```python
from build123d import *

# Parameters (mm, degrees)
BASE_FLANGE1_DEPTH           = 2.65684
SKETCHED_BEND3_DEPTH         = 355.6
SKETCHED_BEND3_2_DEPTH       = 355.6
SKETCH10_R                   = 6.35
CUT_EXTRUDE2_DEPTH           = 2.65684
EDGE_FLANGE5_DEPTH           = 254
EDGE_FLANGE6_STRIP_W         = 16.97736
EDGE_FLANGE6_STRIP_H         = 2.65684
EDGE_FLANGE6_STRIP_CUT_DEPTH = 116.5225
EDGE_FLANGE6_DEPTH           = 116.5225
EDGE_FLANGE7_DEPTH           = 248.16816
SKETCH38_R                   = 2.032
CUT_EXTRUDE4_DEPTH           = 2.65684
SKETCH39_R                   = 2.032
CUT_EXTRUDE5_DEPTH           = 2.65684
SKETCH40_R                   = 6.35
CUT_EXTRUDE6_DEPTH           = 2.65684


# Read off the part's stored shape, not the designer's step: Sketched Bend3
# Sheet-metal steps are written as plain solids
with BuildPart() as part:
    # Sketch1 → Base-Flange1 (new body)
    with BuildSketch(Plane.XY):
        with BuildLine():
            Line((0, 0), (0, 254))
            Line((0, 254), (165.1, 254))
            ThreePointArc((165.1, 254), (177.8, 241.3), (190.5, 254))
            Line((190.5, 254), (355.6, 254))
            Line((355.6, 254), (355.6, 0))
            Line((355.6, 0), (355.6, -57.15))
            Line((355.6, -57.15), (0, -57.15))
            Line((0, -57.15), (0, 0))
        make_face()
    extrude(amount=-BASE_FLANGE1_DEPTH)

    # Sketched Bend3 outline → Sketched Bend3 (cut)
    with BuildSketch(Plane.YZ):
        with BuildLine():
            ThreePointArc((0, -2.65684), (-2.783367186, -1.949765838), (-4.891802611, 0))
            Line((-4.891802611, 0), (-57.15, 0))
            Line((-57.15, 0), (-57.15, -2.65684))
            Line((-57.15, -2.65684), (0, -2.65684))
        make_face()
    extrude(amount=SKETCHED_BEND3_DEPTH, mode=Mode.SUBTRACT)

    # Sketched Bend3 2 outline → Sketched Bend3 2 (add)
    with BuildSketch(Plane.YZ):
        with BuildLine():
            ThreePointArc((0, 0), (-2.24506403, 0.92993597), (-3.175, 3.175))
            Line((-3.175, 3.175), (-3.175, 53.251044406))
            Line((-3.175, 53.251044406), (-5.83184, 53.251044406))
            Line((-5.83184, 53.251044406), (-5.83184, 3.175))
            ThreePointArc((-5.83184, 3.175), (-5.591894488, 1.519381136), (-4.891802611, 0))
            Line((-4.891802611, 0), (0, 0))
        make_face()
    extrude(amount=SKETCHED_BEND3_2_DEPTH)

    # Sketch10 → Cut-Extrude2 (cut)
    with BuildSketch(Plane(origin=(0, -3.175, 0), x_dir=(1, 0, 0), z_dir=(0, 1, 0))):
        with Locations(Location((317.5, -34.201044406, 0), (0, 0, 270))):
            Circle(SKETCH10_R)
        with Locations(Location((247.65, -34.201044406, 0), (0, 0, 270))):
            Circle(SKETCH10_R)
        with Locations(Location((38.1, -34.201044406, 0), (0, 0, 270))):
            Circle(SKETCH10_R)
        with Locations(Location((107.95, -34.201044406, 0), (0, 0, 270))):
            Circle(SKETCH10_R)
        with Locations(Location((177.8, -34.201044406, 0), (0, 0, 270))):
            Circle(SKETCH10_R)
    extrude(amount=-CUT_EXTRUDE2_DEPTH, mode=Mode.SUBTRACT)

    # Edge-Flange5 section (across the edge) → Edge-Flange5 (add)
    with BuildSketch(Plane(origin=(-3.175, 0, -2.65684), x_dir=(1, 0, 0), z_dir=(0, 1, 0))):
        with BuildLine():
            Line((-2.65684, 3.175), (-2.65684, 119.6975))
            Line((-2.65684, 119.6975), (0, 119.6975))
            Line((0, 119.6975), (0, 3.175))
            ThreePointArc((0, 3.175), (0.92993597, 0.92993597), (3.175, 0))
            Line((3.175, 0), (3.175, -2.65684))
            ThreePointArc((3.175, -2.65684), (-0.948733611, -0.948733611), (-2.65684, 3.175))
        make_face()
    extrude(amount=EDGE_FLANGE5_DEPTH)

    # Edge-Flange6 strip (across the edge) → Edge-Flange6 strip cut (cut)
    with BuildSketch(Plane(origin=(-5.83184, 254, -5.83184), x_dir=(0, -1, 0), z_dir=(0, 0, -1))):
        with Locations((-2.65684, -1.32842)):
            Rectangle(EDGE_FLANGE6_STRIP_W, EDGE_FLANGE6_STRIP_H)
    extrude(amount=EDGE_FLANGE6_STRIP_CUT_DEPTH, mode=Mode.SUBTRACT)

    # Edge-Flange6 section (across the edge) → Edge-Flange6 (add)
    with BuildSketch(Plane(origin=(-5.83184, 254, -5.83184), x_dir=(0, -1, 0), z_dir=(0, 0, -1))):
        with BuildLine():
            Line((0, 3.175), (0, 53.975))
            Line((0, 53.975), (2.65684, 53.975))
            Line((2.65684, 53.975), (2.65684, 3.175))
            ThreePointArc((2.65684, 3.175), (3.58677597, 0.92993597), (5.83184, 0))
            Line((5.83184, 0), (5.83184, -2.65684))
            ThreePointArc((5.83184, -2.65684), (1.708106389, -0.948733611), (0, 3.175))
        make_face()
    extrude(amount=EDGE_FLANGE6_DEPTH)

    # Edge-Flange7 section (across the edge) → Edge-Flange7 (add)
    with BuildSketch(Plane(origin=(-3.175, 0, -125.52934), x_dir=(0, 0, 1), z_dir=(0, 1, 0))):
        with BuildLine():
            Line((-2.65684, 3.175), (-2.65684, 25.4))
            Line((-2.65684, 25.4), (0, 25.4))
            Line((0, 25.4), (0, 3.175))
            ThreePointArc((0, 3.175), (0.92993597, 0.92993597), (3.175, 0))
            Line((3.175, 0), (3.175, -2.65684))
            ThreePointArc((3.175, -2.65684), (-0.948733611, -0.948733611), (-2.65684, 3.175))
        make_face()
    extrude(amount=EDGE_FLANGE7_DEPTH)

    # Sketch38 → Cut-Extrude4 (cut)
    with BuildSketch(Plane(origin=(0, 0, -128.18618), x_dir=(-1, 0, 0), z_dir=(0, 0, -1))):
        with Locations((-15.875, 239.27816)):
            Circle(SKETCH38_R)
        with Locations((-15.875, 213.87816)):
            Circle(SKETCH38_R)
        with Locations((-15.875, 188.47816)):
            Circle(SKETCH38_R)
        with Locations((-15.875, 163.07816)):
            Circle(SKETCH38_R)
        with Locations((-15.875, 137.67816)):
            Circle(SKETCH38_R)
        with Locations((-15.875, 112.27816)):
            Circle(SKETCH38_R)
        with Locations((-15.875, 86.87816)):
            Circle(SKETCH38_R)
        with Locations((-15.875, 61.47816)):
            Circle(SKETCH38_R)
        with Locations((-15.875, 36.07816)):
            Circle(SKETCH38_R)
        with Locations((-15.875, 10.67816)):
            Circle(SKETCH38_R)
    extrude(amount=-CUT_EXTRUDE4_DEPTH, mode=Mode.SUBTRACT)

    # Sketch39 → Cut-Extrude5 (cut)
    with BuildSketch(Plane.XY):
        with Locations((339.725, 10.67816)):
            Circle(SKETCH39_R)
        with Locations((339.725, 36.07816)):
            Circle(SKETCH39_R)
        with Locations((339.725, 61.47816)):
            Circle(SKETCH39_R)
        with Locations((339.725, 86.87816)):
            Circle(SKETCH39_R)
        with Locations((339.725, 112.27816)):
            Circle(SKETCH39_R)
        with Locations((339.725, 137.67816)):
            Circle(SKETCH39_R)
        with Locations((339.725, 163.07816)):
            Circle(SKETCH39_R)
        with Locations((339.725, 188.47816)):
            Circle(SKETCH39_R)
        with Locations((339.725, 213.87816)):
            Circle(SKETCH39_R)
        with Locations((339.725, 239.27816)):
            Circle(SKETCH39_R)
    extrude(amount=-CUT_EXTRUDE5_DEPTH, mode=Mode.SUBTRACT)

    # Sketch40 → Cut-Extrude6 (cut)
    with BuildSketch(Plane.ZY.offset(5.83184)):
        with Locations((-34.40684, 41.79316)):
            Circle(SKETCH40_R)
        with Locations((-90.28684, 41.79316)):
            Circle(SKETCH40_R)
    extrude(amount=-CUT_EXTRUDE6_DEPTH, mode=Mode.SUBTRACT)


solid = part.part
```
Model file for the job. Use its own axes, mm. A direction names the side the tool comes from. Give positions to 0.01 mm unless a question says otherwise; leave off trailing zeros. Loops run counter-clockwise (first coordinate to the right, second up) from the corner with the lowest first, then second, coordinate; pieces in that order, holes last. Notation, with made-up numbers: (78, -35.5) -> (118, -35.5) arc R12 cw to (118, -12.5) -> close; hole circle Ø9 at (-24, -16). An arc over 180 degrees is marked (long way). Use CSV: the item, a comma, the result in double quotes. Start each with the question number.
1) Slice it at C-C on z = -49. Give the cut face in (x, y) (3 decimals).
2) Wall check: line 1 (Z direction, x = 235, y = 46); line 2 (Y direction, x = -28.5, z = -69); line 3 (Y direction, x = 238.5, z = 41) (3 decimals). Give the ranges that are in metal, low to high.
3) Flat gauge pins, fed straight in: pin 1 Ø7.5 at (y, z) = (41.79, -90.29) entering from +X; pin 2 Ø1.5 at (y, z) = (204.5, -75) entering from +X (3 decimals); pin 3 Ø2 at (x, z) = (67.5, 25.5) entering from +Y (3 decimals); pin 4 Ø1.5 at (x, y) = (-4.5, 130) entering from +Z. Where does each tip first touch, or does it go through?
4) Slice it at D-D on x = 58.5. Give the cut face in (y, z) (3 decimals).
5) Mould opens along Y. For faces 1 (the cylindrical face through (35.668, -4.485, 40.067)), 2 (the cylindrical face through (-4.52, 48.09, -91.11)), 3 (the flat face through (175, -3.175, 28)), 4 (the flat face through (-35, 251.343, -63)) say: released by +Y, released by -Y, zero draft, split by the parting line, or undercut.
6) Slice it at B-B on y = 173. Give the cut face in (x, z) (3 decimals), plus the area to 3 significant figures.
7) Tool access for faces 5 (the flat face through (-3.175, 122, -65)), 6 (the flat face through (-5.832, 122, -63)), 7 (the flat face through (180, 129, 0)): list every direction of +Z, -Z, +X, -X, +Y, -Y with a clear straight run to the whole face (end or side of a thin tool).
8) Slice it at A-A on x = 107.95. Give the cut face in (y, z) (3 decimals).
Computed values:
1,outline,"(-59.807, 251.343) -> (-9.007, 251.343) arc R3.175 cw to (-5.832, 248.168) -> (-5.832, 0) -> (-3.175, 0) -> (-3.175, 248.168) arc R5.832 ccw to (-9.007, 254) -> (-59.807, 254) -> close"
2,line 1,"z = -2.66 to 0"
2,line 2,"y = 251.34 to 254"
2,line 3,"y = -5.832 to -3.175"
3,pin 1,"passes through"
3,pin 2,"stops at x = -3.175"
3,pin 3,"stops at y = -3.175"
3,pin 4,"stops at z = -1.37"
4,outline,"(-5.832, 3.175) arc R5.832 ccw to (0, -2.657) -> (254, -2.657) -> (254, 0) -> (0, 0) arc R3.175 cw to (-3.175, 3.175) -> (-3.175, 53.251) -> (-5.832, 53.251) -> close"
5,face 1,"zero draft"
5,face 2,"undercut"
5,face 3,"released by +Y"
5,face 4,"released by -Y"
6,outline,"(-5.832, -122.354) arc R5.832 ccw to (0, -128.186) -> (22.225, -128.186) -> (22.225, -125.529) -> (0, -125.529) arc R3.175 cw to (-3.175, -122.354) -> (-3.175, -5.832) arc R3.175 cw to (0, -2.657) -> (355.6, -2.657) -> (355.6, 0) -> (0, 0) arc R5.832 ccw to (-5.832, -5.832) -> close"
6,area,"1,350 mm^2"
7,face 5,"+X, +Y, -Y"
7,face 6,"+Z, -Z, -X, -Y"
7,face 7,"+Z, +X, -X, +Y"
8,outline,"(-5.832, 3.175) arc R5.832 ccw to (0, -2.657) -> (254, -2.657) -> (254, 0) -> (0, 0) arc R3.175 cw to (-3.175, 3.175) -> (-3.175, 27.851) -> (-5.832, 27.851) -> close; (-5.832, 40.551) -> (-3.175, 40.551) -> (-3.175, 53.251) -> (-5.832, 53.251) -> close"
